Work out the finished part from the listing and answer in its coordinate system (mm). Face numbers are marked on the shaded views. Coordinates: 2 decimals unless noted, no trailing zeros. Order: outer loops, then holes, each group sorted by start corner. A loop starts at its lowest first (then second) coordinate and runs counter-clockwise, first axis right, second up. Notation, with made-up numbers: M 24.25,49.5 L 45.25,49.5 A21 cw 45.25,78.5 Z; hole C -5.75,18 d1. An arc over 180 degrees is marked long. Use a Markdown table: item, result.
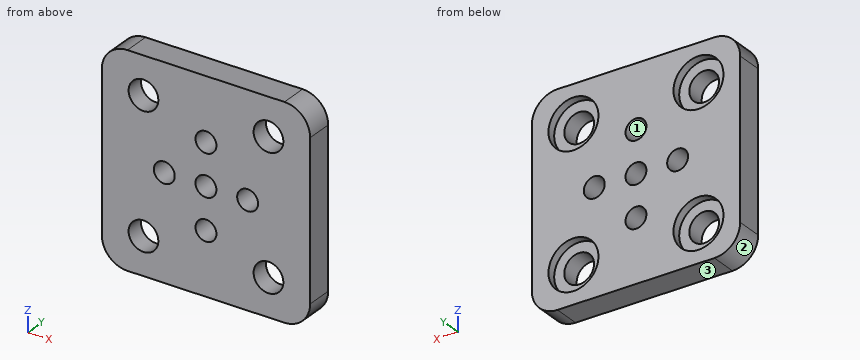
from build123d import *

# Parameters (mm, degrees)
F0_R     = 6
F0_R_2   = 2.51
F0_R_3   = 3.57
F1_DEPTH = 6.35
F2_DEPTH = 2


with BuildPart() as f1:
    # F0 (on Front) → F1 (new body)
    with BuildSketch(Plane.XZ):
        with BuildLine():
            Line((-18.83, -25), (18.83, -25))
            ThreePointArc((18.83, -25), (23.192849, -23.192849), (25, -18.83))
            Line((25, -18.83), (25, 18.83))
            ThreePointArc((25, 18.83), (23.192849, 23.192849), (18.83, 25))
            Line((18.83, 25), (-18.83, 25))
            ThreePointArc((-18.83, 25), (-23.192849, 23.192849), (-25, 18.83))
            Line((-25, 18.83), (-25, -18.83))
            ThreePointArc((-25, -18.83), (-23.192849, -23.192849), (-18.83, -25))
        make_face()
        with Locations((-14.999998, -15.950001)):
            Circle(F0_R, mode=Mode.SUBTRACT)
        with Locations((14.999999, -15.95)):
            Circle(F0_R, mode=Mode.SUBTRACT)
        with Locations((0, -10)):
            Circle(F0_R_2, mode=Mode.SUBTRACT)
        with Locations((-10, 0)):
            Circle(F0_R_2, mode=Mode.SUBTRACT)
        with Locations((-1e-06, 10)):
            Circle(F0_R_2, mode=Mode.SUBTRACT)
        with Locations((-15.000001, 15.949999)):
            Circle(F0_R, mode=Mode.SUBTRACT)
        Circle(F0_R_2, mode=Mode.SUBTRACT)
        with Locations((10, 0)):
            Circle(F0_R_2, mode=Mode.SUBTRACT)
        with Locations((14.999999, 15.95)):
            Circle(F0_R, mode=Mode.SUBTRACT)
        with Locations((-15.000001, 15.949999)):
            Circle(F0_R)
        with Locations((-15.000001, 15.949999)):
            Circle(F0_R_3, mode=Mode.SUBTRACT)
        with Locations((14.999999, 15.95)):
            Circle(F0_R)
        with Locations((14.999999, 15.95)):
            Circle(F0_R_3, mode=Mode.SUBTRACT)
        with Locations((14.999999, -15.95)):
            Circle(F0_R)
        with Locations((14.999999, -15.95)):
            Circle(F0_R_3, mode=Mode.SUBTRACT)
        with Locations((-14.999998, -15.950001)):
            Circle(F0_R)
        with Locations((-14.999998, -15.950001)):
            Circle(F0_R_3, mode=Mode.SUBTRACT)
    extrude(amount=F1_DEPTH)

    # F0 (on Front) → F2 (cut)
    with BuildSketch(Plane.XZ):
        with Locations((14.999999, 15.95)):
            Circle(F0_R)
        with Locations((14.999999, 15.95)):
            Circle(F0_R_3, mode=Mode.SUBTRACT)
        with Locations((-15.000001, 15.949999)):
            Circle(F0_R)
        with Locations((-15.000001, 15.949999)):
            Circle(F0_R_3, mode=Mode.SUBTRACT)
        with Locations((-14.999998, -15.950001)):
            Circle(F0_R)
        with Locations((-14.999998, -15.950001)):
            Circle(F0_R_3, mode=Mode.SUBTRACT)
        with Locations((14.999999, -15.95)):
            Circle(F0_R)
        with Locations((14.999999, -15.95)):
            Circle(F0_R_3, mode=Mode.SUBTRACT)
    extrude(amount=F2_DEPTH, mode=Mode.SUBTRACT)


solid = f1.part
1. Section D-D on z = 9 is taken. Determine the outline of the cut face in (x, y), then the cut area to 3 significant figures.
Answers below:
| item | result |
|---|---|
| outline | M -25,-6.35 L -2.3,-6.35 L -2.3,0 L -25,0 Z; M 2.3,-6.35 L 25,-6.35 L 25,0 L 2.3,0 Z |
| area | 288 mm² |
2. Section A-A on y = -5 is taken. Give the number of separate pieces and of enclosed holes in the cut face, then the cut area to 3 significant figures.
Answers below:
| item | result |
|---|---|
| separate pieces | 1 |
| enclosed holes | 9 |
| area | 2,210 mm² |
3. Find the intervals of material crossed by probe 1 along Z at (x, y) = (0, -4.5); probe 2 along Z at (x, y) = (15, -0.5); probe 3 along X at (y, z) = (-0.25, -11), in increasing order.
Answers below:
| item | result |
|---|---|
| probe 1 | -25 to -12.51, -7.49 to -2.51, 2.51 to 7.49, 12.51 to 25 |
| probe 2 | -25 to -21.95, -9.95 to 9.95, 21.95 to 25 |
| probe 3 | -25 to -18.39, -11.61 to -2.3, 2.3 to 11.61, 18.39 to 25 |
4. Section B-B on z = 15.95 is taken. Determine the outline of the cut face in (x, y), then the cut area to 3 significant figures.
Answers below:
| item | result |
|---|---|
| outline | M -25,-6.35 L -18.57,-6.35 L -18.57,-2 L -21,-2 L -21,0 L -25,0 Z; M -11.43,-6.35 L 11.43,-6.35 L 11.43,-2 L 9,-2 L 9,0 L -9,0 L -9,-2 L -11.43,-2 Z; M 18.57,-6.35 L 25,-6.35 L 25,0 L 21,0 L 21,-2 L 18.57,-2 Z |
| area | 207 mm² |
5. For a pull along X with two mould halves and no side action, classify the marked faces 1, 2 and 3 as +X half, -X half, draft (parallel to the pull), parting line (faces both ways), or undercut.
Answers below:
| item | result |
|---|---|
| face 1 | undercut |
| face 2 | -X half |
| face 3 | draft |
6. Section C-C on x = -18 is taken. Determine the outline of the cut face in (y, z).
Answers below:
| item | result |
|---|---|
| outline | M -6.35,-25 L 0,-25 L 0,-21.15 L -2,-21.15 L -2,-17.89 L -6.35,-17.89 Z; M -6.35,-14.01 L -2,-14.01 L -2,-10.75 L 0,-10.75 L 0,10.75 L -2,10.75 L -2,14.01 L -6.35,14.01 Z; M -6.35,17.89 L -2,17.89 L -2,21.15 L 0,21.15 L 0,25 L -6.35,25 Z |
7. Flat-ended cylindrical pins translate along their axes: P1, Ø9.5, axis at x = 15, z = -15.95, coming from the +Y side; P2, Ø4, axis at x = 10, z = 0, coming from the -Y side. Find the tip coordinate at first contact, or state that the pin passes through.
Answers below:
| item | result |
|---|---|
| P1 | y = -2 |
| P2 | through |
